For this review, take the finished solid that the model builds, in its own axes (mm). Face numbers are marked on the shaded views. A direction names the side the tool comes from. Coordinates: 2 decimals unless noted, no trailing zeros. Loops run counter-clockwise (first coordinate to the right, second up) from the corner with the lowest first, then second, coordinate; pieces in that order, holes last. Notation, with made-up numbers: (70.5, -16.75) -> (84.5, -16.75) arc R9 ccw to (84.5, -9.75) -> close; hole circle Ø6 at (14.25, 9.25). An arc over 180 degrees is marked (long way). Use a Markdown table: item, result.
from build123d import *

# Parameters (mm, degrees)
SKETCH_R      = 2.25
PAD_DEPTH     = 4
SKETCH001_R   = 5
SKETCH001_R_2 = 2.25
PAD001_DEPTH  = 4
SKETCH004_R   = 4
SKETCH004_R_2 = 2.25
PAD004_DEPTH  = 8


with BuildPart() as part:
    # Sketch → Pad (new body)
    with BuildSketch(Plane.XZ):
        Polygon((7, 0), (3.5, 6.062178), (-3.5, 6.062178), (-7, 0), (-3.5, -6.062178), (3.5, -6.062178), align=None)
        Circle(SKETCH_R, mode=Mode.SUBTRACT)
    extrude(amount=PAD_DEPTH)

    # Sketch001 (on Face9 of Pad) → Pad001 (join)
    with BuildSketch(Plane.XZ.offset(4)):
        Circle(SKETCH001_R)
        Circle(SKETCH001_R_2, mode=Mode.SUBTRACT)
    extrude(amount=PAD001_DEPTH)

    # Sketch004 (on Face12 of Pad001) → Pad004 (join)
    with BuildSketch(Plane.XZ.offset(8)):
        Circle(SKETCH004_R)
        Circle(SKETCH004_R_2, mode=Mode.SUBTRACT)
    extrude(amount=PAD004_DEPTH)


with BuildPart() as part_1:
    # Body placement: moved
    add(part.part.moved(Location((20, 168, 61))))


solid = part_1.part
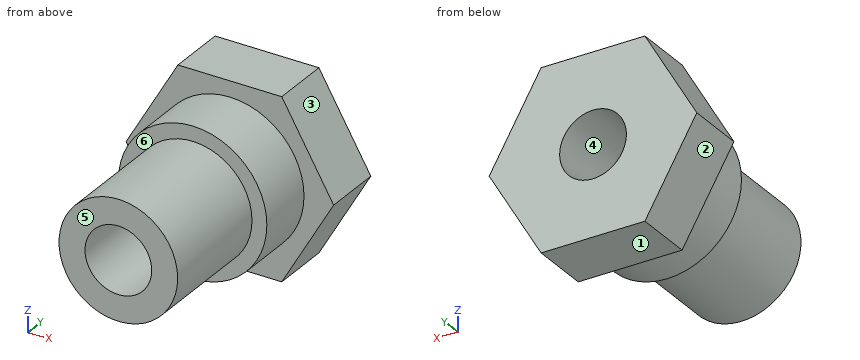
(1) Take a section at B-B on y = 166.5. Write out the cut boundary in (x, z).
Found:
| item | result |
|---|---|
| outline | (13, 61) -> (16.5, 54.94) -> (23.5, 54.94) -> (27, 61) -> (23.5, 67.06) -> (16.5, 67.06) -> close; hole circle Ø4.5 at (20, 61) |
(2) For pin 1 Ø4 at (x, y) = (24.5, 158) entering from +Z; pin 2 Ø5 at (x, y) = (20, 155.5) entering from +Z; pin 3 Ø5 at (y, z) = (156, 61.5) entering from -X, all flat-tipped, find the tip position at first contact; note any pin that passes through.
Found:
| item | result |
|---|---|
| pin 1 | stops at z = 64.12 |
| pin 2 | stops at z = 65 |
| pin 3 | stops at x = 16 |
(3) For line 1 along Z through (x, y) = (20, 163.75); line 2 along Z through (x, y) = (20, 154.5); line 3 along Y through (x, z) = (16.5, 65.75), list the stretches that pass through material, from the lowest coordinate up.
Found:
| item | result |
|---|---|
| line 1 | z = 56 to 58.75, 63.25 to 66 |
| line 2 | z = 57 to 58.75, 63.25 to 65 |
| line 3 | y = 164 to 168 |
(4) Take a section at A-A on x = 20. Write out the cut boundary in (y, z).
Found:
| item | result |
|---|---|
| outline | (152, 57) -> (160, 57) -> (160, 56) -> (164, 56) -> (164, 54.94) -> (168, 54.94) -> (168, 58.75) -> (152, 58.75) -> close; (152, 63.25) -> (168, 63.25) -> (168, 67.06) -> (164, 67.06) -> (164, 66) -> (160, 66) -> (160, 65) -> (152, 65) -> close |
(5) Take a section at C-C on z = 61.5. Write out the cut boundary in (x, y), plus the area to 3 significant figures.
Found:
| item | result |
|---|---|
| outline | (13.29, 164) -> (15.03, 164) -> (15.03, 160) -> (16.03, 160) -> (16.03, 152) -> (17.81, 152) -> (17.81, 168) -> (13.29, 168) -> close; (22.19, 152) -> (23.97, 152) -> (23.97, 160) -> (24.97, 160) -> (24.97, 164) -> (26.71, 164) -> (26.71, 168) -> (22.19, 168) -> close |
| area | 86.8 mm^2 |
(6) Mouldability with a two-part tool opening along X and no side actions: class the marked faces 1, 2, 3 and 4 as pulls with the +X half, pulls with the -X half, needs draft (parallel to the pull), parting line crosses it, or undercut.
Found:
| item | result |
|---|---|
| face 1 | needs draft |
| face 2 | pulls with the -X half |
| face 3 | pulls with the +X half |
| face 4 | undercut |
(7) For the marked faces 5 and 6, list the 3-axis set-ups (+Z, -Z, +X, -X, +Y, -Y) from which the entire face can be reached by the end or side of a thin tool; tool diameter is ignored.
Found:
| item | result |
|---|---|
| face 5 | +Z, -Z, +X, -X, -Y |
| face 6 | -Y |
(8) Take a section at D-D on z = 64. Write out the cut boundary in (x, y), plus the area to 3 significant figures.
Found:
| item | result |
|---|---|
| outline | (14.73, 164) -> (16, 164) -> (16, 160) -> (17.35, 160) -> (17.35, 152) -> (22.65, 152) -> (22.65, 160) -> (24, 160) -> (24, 164) -> (25.27, 164) -> (25.27, 168) -> (14.73, 168) -> close |
| area | 116 mm^2 |
